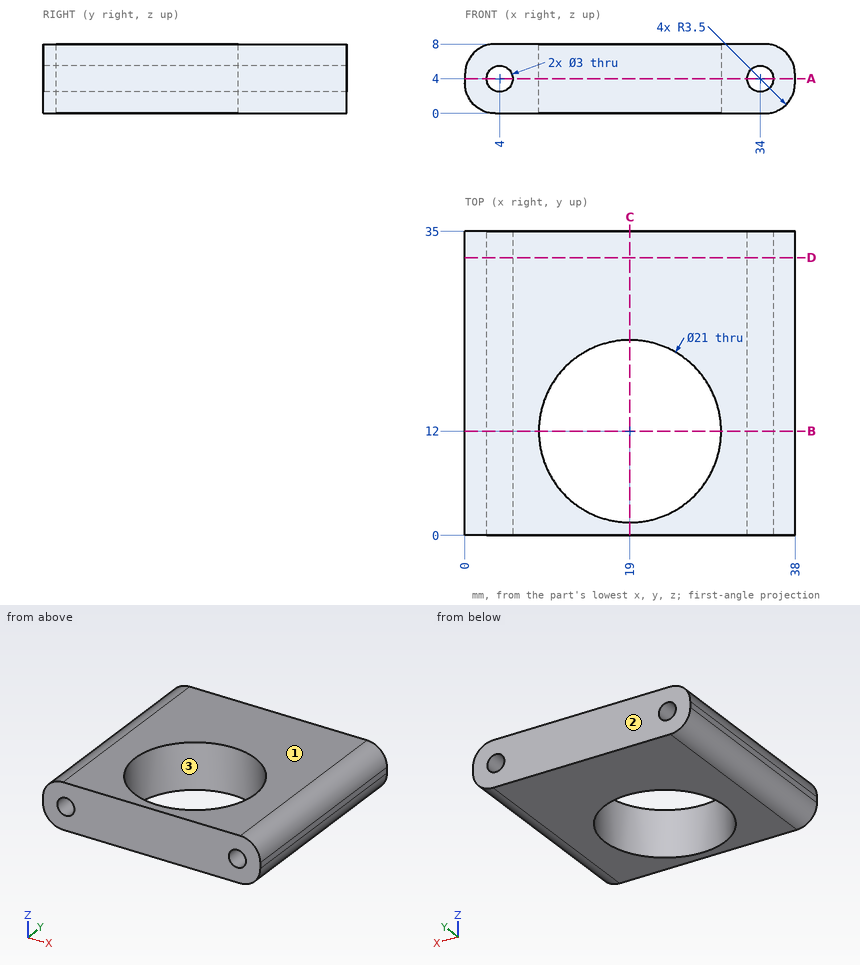
For this review, use the dimensioned drawing (mm, ordinates from the lowest corner) and the shaded views. Give positions to 0.01 mm unless a question says otherwise; leave off trailing zeros. Loops run counter-clockwise (first coordinate to the right, second up) from the corner with the lowest first, then second, coordinate; pieces in that order, holes last. Notation, with made-up numbers: (-11.5, -32) -> (25.5, -32) arc R13 cw to (25.5, -28) -> close; hole circle Ø6 at (-21, 56). An arc over 180 degrees is marked (long way). One line per question, with ' | ' between items. Start each with the question number.
(1) Insertion check: P1, Ø4, axis at x = 21.5, z = 3.5, coming from the -Y side. The pin has a flat end and moves straight along its axis. Give the tip position at first contact, or say it passes through.
(2) For line 1 (Y direction, x = 19, z = 2.25); line 2 (X direction, y = 20.5, z = 3); line 3 (X direction, y = 14, z = 5.25), list the stretches that pass through material, from the lowest coordinate up.
(3) We need section A-A (z = 4). State the section outline as (x, y) points, and give its area (3 significant figures).
(4) We need section D-D (y = 32). State the section outline as (x, z) points.
(5) We need section B-B (y = 12). State the section outline as (x, z) points.
(6) We need section C-C (x = 19). State the section outline as (y, z) points, and give its area (3 significant figures).
(7) Draft analysis for pull direction Y (two halves, no side actions). For the marked faces 1, 2 and 3, state which applies: +Y half, -Y half, draft (parallel to the pull), parting line (faces both ways), or undercut.
The answers:
1) P1: stops at y = 0
2) line 1: y = 0 to 1.5, 22.5 to 35 | line 2: x = 0.04 to 2.88, 5.12 to 12.84, 25.16 to 32.88, 35.12 to 37.96 | line 3: x = 0.08 to 3.17, 4.83 to 8.69, 29.31 to 33.17, 34.83 to 37.92
3) outline: (0, 0) -> (2.5, 0) -> (2.5, 35) -> (0, 35) -> close; (5.5, 0) -> (32.5, 0) -> (32.5, 35) -> (5.5, 35) -> close; (35.5, 0) -> (38, 0) -> (38, 35) -> (35.5, 35) -> close; hole circle Ø21 at (19, 12) | area: 774 mm^2
4) outline: (0, 3.5) arc R3.5 ccw to (3.5, 0) -> (34.5, 0) arc R3.5 ccw to (38, 3.5) -> (38, 4.5) arc R3.5 ccw to (34.5, 8) -> (3.5, 8) arc R3.5 ccw to (0, 4.5) -> close; hole circle Ø3 at (4, 4); hole circle Ø3 at (34, 4)
5) outline: (0, 3.5) arc R3.5 ccw to (3.5, 0) -> (8.5, 0) -> (8.5, 8) -> (3.5, 8) arc R3.5 ccw to (0, 4.5) -> close; (29.5, 0) -> (34.5, 0) arc R3.5 ccw to (38, 3.5) -> (38, 4.5) arc R3.5 ccw to (34.5, 8) -> (29.5, 8) -> close; hole circle Ø3 at (4, 4); hole circle Ø3 at (34, 4)
6) outline: (0, 0) -> (1.5, 0) -> (1.5, 8) -> (0, 8) -> close; (22.5, 0) -> (35, 0) -> (35, 8) -> (22.5, 8) -> close | area: 112 mm^2
7) face 1: draft | face 2: +Y half | face 3: undercut
